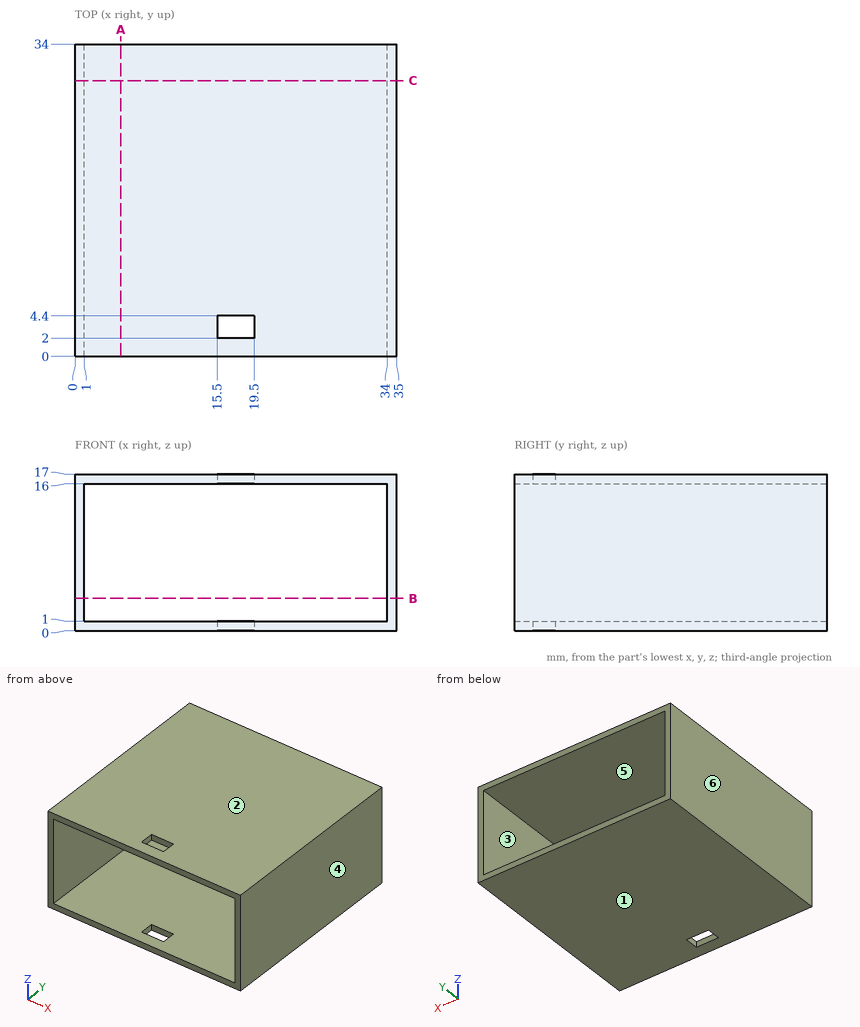
Could you check a few things on this drawing? It's one solid part, dimensions in mm from its lowest x, y, z. A direction names the side the tool comes from. Give positions to 0.01 mm unless a question says otherwise; leave off trailing zeros. Loops run counter-clockwise (first coordinate to the right, second up) from the corner with the lowest first, then second, coordinate; pieces in that order, holes last. Notation, with made-up numbers: (39, 42) -> (74, 42) arc R20 ccw to (74, 71) -> close; hole circle Ø9 at (22.5, -27). An arc over 180 degrees is marked (long way). Answer as CSV lines item,"result". Start each with the question number.
(1) If we section it at C-C on y = 30: Write out the boundary of the cut face in (x, z).
(2) Which directions (+Z, -Z, +X, -X, +Y, -Y) give clear straight access to the entire face, cutting with the end or side of a thin tool? Please do the marked faces 5 and 6.
(3) We'd pull the mould along Z, two halves only. Please class the marked faces 1, 2, 3 and 4: released by +Z, released by -Z, zero draft, split by the parting line, or undercut.
(4) I need wall thicknesses on probe 1 along X at (y, z) = (5, 4.25); probe 2 along Z at (x, y) = (9, 18.5). Which ranges of each line are inside material? Lowest first, please.
(5) If we section it at B-B on z = 3.5: Write out the boundary of the cut face in (x, y).
(6) If we section it at A-A on x = 5: Write out the boundary of the cut face in (y, z).
Computed:
1,outline,"(0, 0) -> (35, 0) -> (35, 17) -> (0, 17) -> close; hole (1, 1) -> (34, 1) -> (34, 16) -> (1, 16) -> close"
2,face 5,"+Y, -Y"
2,face 6,"+Z, -Z, -X, +Y, -Y"
3,face 1,"released by -Z"
3,face 2,"released by +Z"
3,face 3,"undercut"
3,face 4,"zero draft"
4,probe 1,"x = 0 to 1, 34 to 35"
4,probe 2,"z = 0 to 1, 16 to 17"
5,outline,"(0, 0) -> (1, 0) -> (1, 34) -> (0, 34) -> close; (34, 0) -> (35, 0) -> (35, 34) -> (34, 34) -> close"
6,outline,"(0, 0) -> (34, 0) -> (34, 1) -> (0, 1) -> close; (0, 16) -> (34, 16) -> (34, 17) -> (0, 17) -> close"
